from build123d import *

# Parameters (mm, degrees)
SKETCH1_R                = 1.5
SKETCH1_R_2              = 11.683085131
BOSS_EXTRUDE1_DEPTH      = 3
SKETCH2_W                = 26.83266495
SKETCH2_H                = 4
BOSS_EXTRUDE2_DEPTH      = 70.321471268
BOSS_EXTRUDE3_DEPTH      = 2
BOSS_EXTRUDE3_DEPTH_BACK = 8
SKETCH4_R                = 1.5
CUT_EXTRUDE1_DEPTH       = 20
CHAMFER1_SIZE            = 1
CHAMFER2_SIZE            = 1
CHAMFER3_SIZE            = 1
CHAMFER4_SIZE            = 0.5


# Some blends are built 0.0001 mm under size
with BuildPart() as part:
    # Sketch1 → Boss-Extrude1 (new body)
    with BuildSketch(Plane.XY):
        with BuildLine():
            Line((20.560660172, 16.939339828), (16.939339828, 20.560660172))
            ThreePointArc((16.939339828, 20.560660172), (16.452704805, 20.885819299), (15.878679656, 21))
            Line((15.878679656, 21), (-15.878679656, 21))
            ThreePointArc((-15.878679656, 21), (-16.452704805, 20.885819299), (-16.939339828, 20.560660172))
            Line((-16.939339828, 20.560660172), (-20.560660172, 16.939339828))
            ThreePointArc((-20.560660172, 16.939339828), (-20.885819299, 16.452704805), (-21, 15.878679656))
            Line((-21, 15.878679656), (-21, -15.878679656))
            ThreePointArc((-21, -15.878679656), (-20.885819299, -16.452704805), (-20.560660172, -16.939339828))
            Line((-20.560660172, -16.939339828), (-16.939339828, -20.560660172))
            ThreePointArc((-16.939339828, -20.560660172), (-16.452704805, -20.885819299), (-15.878679656, -21))
            Line((-15.878679656, -21), (15.878679656, -21))
            ThreePointArc((15.878679656, -21), (16.452704805, -20.885819299), (16.939339828, -20.560660172))
            Line((16.939339828, -20.560660172), (20.560660172, -16.939339828))
            ThreePointArc((20.560660172, -16.939339828), (20.885819299, -16.452704805), (21, -15.878679656))
            Line((21, -15.878679656), (21, 15.878679656))
            ThreePointArc((21, 15.878679656), (20.885819299, 16.452704805), (20.560660172, 16.939339828))
        make_face()
        with Locations((-15.5, 15.5)):
            Circle(SKETCH1_R, mode=Mode.SUBTRACT)
        with Locations((15.5, 15.5)):
            Circle(SKETCH1_R, mode=Mode.SUBTRACT)
        with Locations((15.5, -15.5)):
            Circle(SKETCH1_R, mode=Mode.SUBTRACT)
        with Locations((-15.5, -15.5)):
            Circle(SKETCH1_R, mode=Mode.SUBTRACT)
        Circle(SKETCH1_R_2, mode=Mode.SUBTRACT)
    extrude(amount=BOSS_EXTRUDE1_DEPTH)

    # Sketch2 → Boss-Extrude2 (add)
    with BuildSketch(Plane.XY.offset(3)):
        with Locations((0, -19)):
            Rectangle(SKETCH2_W, SKETCH2_H)
        with Locations((0, 19)):
            Rectangle(SKETCH2_W, SKETCH2_H)
    extrude(amount=BOSS_EXTRUDE2_DEPTH)

    # Sketch3 → Boss-Extrude3 (add, two sides: drawn at the far end of the back side and taken through both)
    with BuildSketch(Plane.XY.offset(73.321471268).offset(-BOSS_EXTRUDE3_DEPTH_BACK)):
        with BuildLine():
            Line((21.416332475, 3.5), (13.416332475, 3.5))
            Line((13.416332475, 3.5), (13.416332475, 21))
            Line((13.416332475, 21), (-13.416332475, 21))
            Line((-13.416332475, 21), (-13.416332475, 3.5))
            Line((-13.416332475, 3.5), (-21.416332475, 3.5))
            Line((-21.416332475, 3.5), (-21.416332475, 0.5))
            Line((-21.416332475, 0.5), (-10.837664512, 0.5))
            ThreePointArc((-10.837664512, 0.5), (-7.492675622, 7.846322966), (0, 10.849192231))
            ThreePointArc((0, 10.849192231), (7.492675622, 7.846322966), (10.837664512, 0.5))
            Line((10.837664512, 0.5), (21.416332475, 0.5))
            Line((21.416332475, 0.5), (21.416332475, 3.5))
        make_face()
        with BuildLine():
            Line((-13.416332475, -21), (13.416332475, -21))
            Line((13.416332475, -21), (13.416332475, -3.5))
            Line((13.416332475, -3.5), (21.416332475, -3.5))
            Line((21.416332475, -3.5), (21.416332475, -0.5))
            Line((21.416332475, -0.5), (10.837664512, -0.5))
            ThreePointArc((10.837664512, -0.5), (0, -10.849192231), (-10.837664512, -0.5))
            Line((-10.837664512, -0.5), (-21.416332475, -0.5))
            Line((-21.416332475, -0.5), (-21.416332475, -3.5))
            Line((-21.416332475, -3.5), (-13.416332475, -3.5))
            Line((-13.416332475, -3.5), (-13.416332475, -21))
        make_face()
    extrude(amount=BOSS_EXTRUDE3_DEPTH + BOSS_EXTRUDE3_DEPTH_BACK)

    # Sketch4 → Cut-Extrude1 (cut)
    with BuildSketch(Plane.XZ.offset(3.5)):
        with Locations((-18.023235698, 72.821471268)):
            Circle(SKETCH4_R)
        with Locations((-18.023235698, 67.821471268)):
            Circle(SKETCH4_R)
        with Locations((18.023235698, 72.821471268)):
            Circle(SKETCH4_R)
        with Locations((18.023235698, 67.821471268)):
            Circle(SKETCH4_R)
    extrude(amount=-CUT_EXTRUDE1_DEPTH, mode=Mode.SUBTRACT)

    # Chamfer1
    chamfer1_edges = [part.edges().sort_by_distance(p)[0] for p in [
        (-13.416332475, 17, 34.160735634),
        (13.416332475, 17, 34.160735634),
        (-13.416332475, -21, 39.160735634),
        (13.416332475, -21, 39.160735634),
        (-13.416332475, 21, 39.160735634),
        (13.416332475, 21, 39.160735634),
        (13.416332475, -17, 34.160735634),
        (-13.416332475, -17, 34.160735634),
    ]]
    chamfer(chamfer1_edges, length=CHAMFER1_SIZE)

    # Chamfer2
    chamfer2_edges = [part.edges().sort_by_distance(p)[0] for p in [
        (-17.416332475, -3.5, 75.321471268),
        (-13.416332475, -10.75, 65.321471268),
        (-17.416332475, -3.5, 65.321471268),
        (-21.416332475, -3.5, 70.321471268),
        (-21.416332475, -2, 75.321471268),
        (-16.126998493, -0.5, 75.321471268),
        (0, -10.849192231, 75.321471268),
        (16.126998493, -0.5, 75.321471268),
        (21.416332475, -2, 75.321471268),
        (-13.416332475, -11.75, 75.321471268),
        (-12.916332475, -20.5, 75.321471268),
        (0, -21, 75.321471268),
        (12.916332475, -20.5, 75.321471268),
        (13.416332475, -11.75, 75.321471268),
        (17.416332475, -3.5, 75.321471268),
        (17.416332475, -3.5, 65.321471268),
        (21.416332475, -3.5, 70.321471268),
        (17.416332475, 3.5, 75.321471268),
        (17.416332475, 3.5, 65.321471268),
        (21.416332475, 3.5, 70.321471268),
        (21.416332475, 2, 75.321471268),
        (16.126998493, 0.5, 75.321471268),
        (0, 10.849192231, 75.321471268),
        (-16.126998493, 0.5, 75.321471268),
        (-21.416332475, 2, 75.321471268),
        (-13.416332475, 10.75, 65.321471268),
        (-17.416332475, 3.5, 65.321471268),
        (-21.416332475, 3.5, 70.321471268),
        (-17.416332475, 3.5, 75.321471268),
        (-13.416332475, 11.75, 75.321471268),
        (-12.916332475, 20.5, 75.321471268),
        (13.416332475, 11.75, 75.321471268),
        (12.916332475, 20.5, 75.321471268),
        (0, 21, 75.321471268),
    ]]
    chamfer(chamfer2_edges, length=CHAMFER2_SIZE - 0.0001)  # a hair under: the kernel refuses the full size

    # Chamfer3
    chamfer3_edges = [part.edges().sort_by_distance(p)[0] for p in [
        (13.416332475, 10.25005, 65.321471268),
        (13.416332475, -10.25005, 65.321471268),
    ]]
    chamfer(chamfer3_edges, length=CHAMFER3_SIZE)

    # Chamfer4
    # the kernel refuses this chamfer: 0.5 mm, written as the material it takes off along each edge
    with BuildSketch(Plane(origin=(-18.023235698, 3.5, 67.821471268), x_dir=(1, 0, 0), z_dir=(0, 0, -1))) as chamfer4_piece_1:
        Polygon((1.5, CHAMFER4_SIZE), (1.5 + CHAMFER4_SIZE, 0), (1.5, 0), align=None)
    revolve(axis=Axis((-18.023235698, 3.5, 67.821471268), (0, -1, 0)), mode=Mode.SUBTRACT)
    with BuildSketch(Plane(origin=(-18.023235698, -3.5, 67.821471268), x_dir=(1, 0, 0), z_dir=(0, 0, -1))) as chamfer4_piece_2:
        Polygon((1.5 + CHAMFER4_SIZE, 0), (1.5, -CHAMFER4_SIZE), (1.5, 0), align=None)
    revolve(axis=Axis((-18.023235698, -3.5, 67.821471268), (0, -1, 0)), mode=Mode.SUBTRACT)
    with BuildSketch(Plane(origin=(18.023235698, -3.5, 72.821471268), x_dir=(1, 0, 0), z_dir=(0, 0, -1))) as chamfer4_piece_3:
        Polygon((1.5 + CHAMFER4_SIZE, 0), (1.5, -CHAMFER4_SIZE), (1.5, 0), align=None)
    revolve(axis=Axis((18.023235698, -3.5, 72.821471268), (0, -1, 0)), mode=Mode.SUBTRACT)
    with BuildSketch(Plane(origin=(18.023235698, 3.5, 72.821471268), x_dir=(1, 0, 0), z_dir=(0, 0, -1))) as chamfer4_piece_4:
        Polygon((1.5 + CHAMFER4_SIZE, 0), (1.5, CHAMFER4_SIZE), (1.5, 0), align=None)
    revolve(axis=Axis((18.023235698, 3.5, 72.821471268), (0, -1, 0)), mode=Mode.SUBTRACT)
    with BuildSketch(Plane(origin=(18.023235698, -3.5, 67.821471268), x_dir=(1, 0, 0), z_dir=(0, 0, -1))) as chamfer4_piece_5:
        Polygon((1.5 + CHAMFER4_SIZE, 0), (1.5, -CHAMFER4_SIZE), (1.5, 0), align=None)
    revolve(axis=Axis((18.023235698, -3.5, 67.821471268), (0, -1, 0)), mode=Mode.SUBTRACT)
    with BuildSketch(Plane(origin=(18.023235698, 3.5, 67.821471268), x_dir=(1, 0, 0), z_dir=(0, 0, -1))) as chamfer4_piece_6:
        Polygon((1.5 + CHAMFER4_SIZE, 0), (1.5, CHAMFER4_SIZE), (1.5, 0), align=None)
    revolve(axis=Axis((18.023235698, 3.5, 67.821471268), (0, -1, 0)), mode=Mode.SUBTRACT)
    with BuildSketch(Plane(origin=(-18.023235698, 3.5, 72.821471268), x_dir=(1, 0, 0), z_dir=(0, 0, -1))) as chamfer4_piece_7:
        Polygon((1.5, CHAMFER4_SIZE), (1.5 + CHAMFER4_SIZE, 0), (1.5, 0), align=None)
    revolve(axis=Axis((-18.023235698, 3.5, 72.821471268), (0, -1, 0)), mode=Mode.SUBTRACT)
    with BuildSketch(Plane(origin=(-18.023235698, -3.5, 72.821471268), x_dir=(1, 0, 0), z_dir=(0, 0, -1))) as chamfer4_piece_8:
        Polygon((1.5 + CHAMFER4_SIZE, 0), (1.5, -CHAMFER4_SIZE), (1.5, 0), align=None)
    revolve(axis=Axis((-18.023235698, -3.5, 72.821471268), (0, -1, 0)), mode=Mode.SUBTRACT)


solid = part.part
Input: part model. Units: mm. Frame: model coordinates. A direction names the side the tool comes from. Coordinates: 2 decimals unless noted, no trailing zeros. Loops run counter-clockwise (first coordinate to the right, second up) from the corner with the lowest first, then second, coordinate; pieces in that order, holes last.
Q1. Set-up query: faces 1 (the face through (-16, 0.5, 70)), 2 (the face through (0.235, -11.006, 74.481)), 3 (the face through (13.416, 18.4, 51.7)). Return all of +Z, -Z, +X, -X, +Y, -Y with unobstructed straight access to the full face (end or side cutting, diameter ignored); none if empty.
Q2. Contact query for flat-ended pins moving along their axis: pin 1 (1.8 mm diameter, centred on x = 18.02, z = 72.82, fed in from -Y); pin 2 (5.5 mm diameter, centred on x = 18, z = 70, fed in from -Y); pin 3 (3 mm diameter, centred on x = -16, y = 8, fed in from +Z); pin 4 (8 mm diameter, centred on y = -15, z = 45.5, fed in from +X). Output: stop coordinate, or through.
Q3. Cut plane B-B (x = -18). Give the number of separate pieces and of enclosed holes in the cut face, then the cut area to 3 significant figures.
Q4. Draft query along Y for faces 4 (the face through (-16, -0.5, 70)), 5 (the face through (-19.214, -1.768, 66.909)), 6 (the face through (-16, -3.5, 70)). Return one class per face: +Y half, -Y half, draft (parallel to the pull), parting line (faces both ways), or undercut.
Q5. Cut plane A-A (z = 5). Output: boundary loops of the cut face in (x, y).
Q6. Material intervals for line 1 (Y direction, x = 15.5, z = 2); line 2 (Y direction, x = -3.5, z = 12); line 3 (Z direction, x = 1, y = 15), sorted ascending.
Working result:
1. face 1: +Z, +X, -X
1. face 2: +Z
1. face 3: +Z, +X, +Y
2. pin 1: passes through
2. pin 2: stops at y = -3.5
2. pin 3: stops at z = 3
2. pin 4: stops at x = 13.42
3. separate pieces: 7
3. enclosed holes: 0
3. area: 137 mm2
4. face 4: undercut
4. face 5: draft
4. face 6: -Y half
5. outline: (-13.42, -20) - (-12.42, -21) - (12.42, -21) - (13.42, -20) - (13.42, -18) - (12.42, -17) - (-12.42, -17) - (-13.42, -18) - close; (-13.42, 18) - (-12.42, 17) - (12.42, 17) - (13.42, 18) - (13.42, 20) - (12.42, 21) - (-12.42, 21) - (-13.42, 20) - close
6. line 1: y = -21 to -17, -14 to 14, 17 to 21
6. line 2: y = -21 to -17, 17 to 21
6. line 3: z = 0 to 3, 65.32 to 75.32
